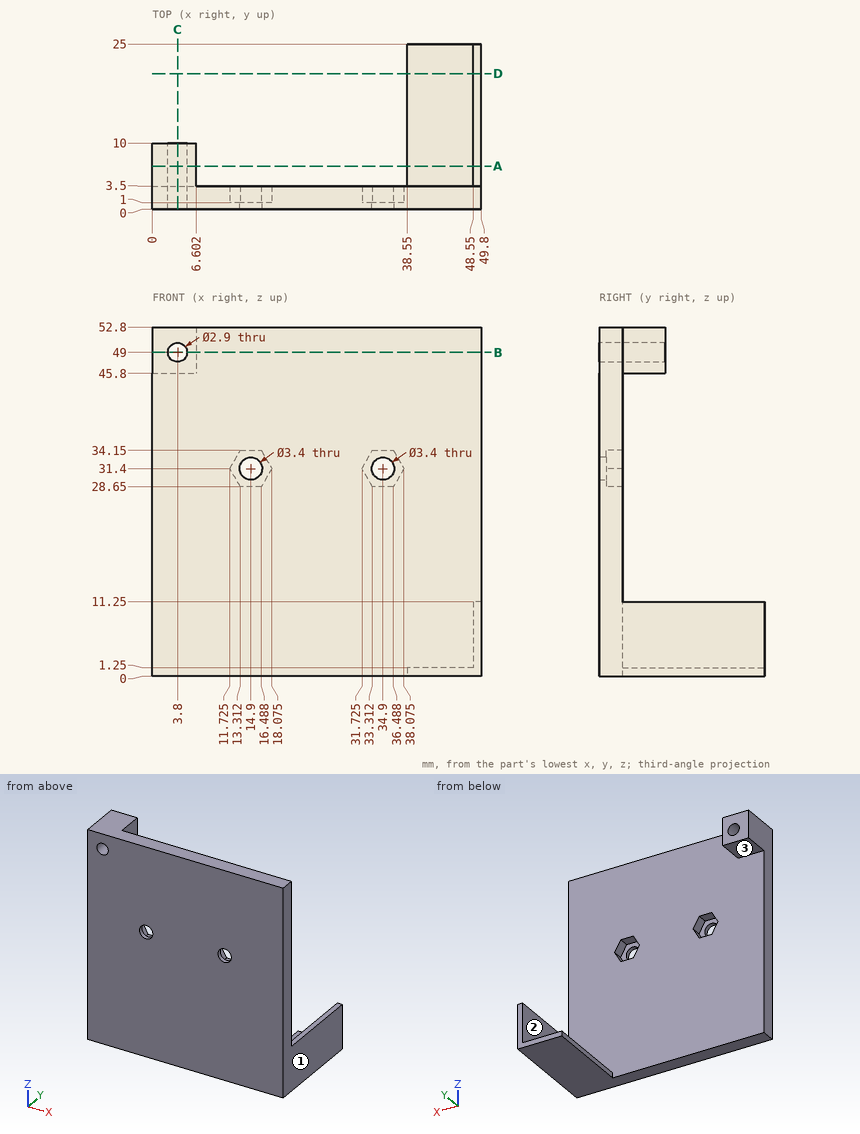
Drawing for the job (mm, zero at the part's lowest x, y, z). A direction names the side the tool comes from. Coordinates: 2 decimals unless noted, no trailing zeros. Write each loop counter-clockwise with the first axis right and the second up, starting at its lowest first coordinate (ties: lowest second). Pieces come first, ordered by that corner, then holes. Notation, with made-up numbers: (64.25, 25) - (80.25, 25) arc R26 ccw to (80.25, 39) - close; hole circle Ø9 at (32.25, 73). An arc over 180 degrees is marked (long way). Write each question's results on one line, items separated by ' | '. Start each with the question number.
1) Probe line 1 along X through (y, z) = (0.7, 31.4); line 2 along Z through (x, y) = (3.8, 7.75); line 3 along Y through (x, z) = (40.5, 18.5). List the from-to ranges inside material, lowest first. Write a range as from..to.
2) Flat gauge pins, fed straight in: P1, Ø0.8, axis at x = 15, y = 2, coming from the -Z side; P2, Ø15, axis at x = 18, z = 19, coming from the +Y side; P3, Ø7.5, axis at x = 2, z = 49, coming from the +Y side; P4, Ø1, axis at x = 49.5, y = 19.5, coming from the +Z side. Where does each tip first touch, or does it go through?
3) Cut at A-A (y = 6.5). Write the cut outline in (x, z).
4) Cut at D-D (y = 20.5). Write the cut outline in (x, z).
5) 3-axis set-ups, long thin cutter, end or side, ignore diameter. For the marked faces 1, 2 and 3: which of +Z, -Z, +X, -X, +Y, -Y reach the whole face in a straight line?
6) Cut at C-C (x = 3.8). Write the cut outline in (y, z).
7) Cut at B-B (z = 49). Write the cut outline in (x, y), then the cut area to 3 significant figures.
Returned:
1) line 1: 0..13.2, 16.6..33.2, 36.6..49.8 | line 2: 45.8..47.55, 50.45..52.8 | line 3: 0..3.5
2) P1: z = 0 | P2: y = 3.5 | P3: y = 10 | P4: z = 11.25
3) outline: (0, 45.8) - (6.6, 45.8) - (6.6, 52.8) - (0, 52.8) - close; (38.55, 0) - (49.8, 0) - (49.8, 11.25) - (48.55, 11.25) - (48.55, 1.25) - (38.55, 1.25) - close; hole circle Ø2.9 at (3.8, 49)
4) outline: (38.55, 0) - (49.8, 0) - (49.8, 11.25) - (48.55, 11.25) - (48.55, 1.25) - (38.55, 1.25) - close
5) face 1: +Z, -Z, +X, +Y, -Y | face 2: +Z, -X, +Y | face 3: -Z, +X, -X, +Y
6) outline: (0, 0) - (3.5, 0) - (3.5, 45.8) - (10, 45.8) - (10, 47.55) - (0, 47.55) - close; (0, 50.45) - (10, 50.45) - (10, 52.8) - (0, 52.8) - close
7) outline: (0, 0) - (2.35, 0) - (2.35, 10) - (0, 10) - close; (5.25, 0) - (49.8, 0) - (49.8, 3.5) - (6.6, 3.5) - (6.6, 10) - (5.25, 10) - close | area: 188 mm^2
